Design review of the part built by this model. Coordinates are the model's own, in mm. A direction names the side the tool comes from. Round coordinates to 2 decimals unless told otherwise and drop trailing zeros. Loops run counter-clockwise (first coordinate to the right, second up) from the corner with the lowest first, then second, coordinate; pieces in that order, holes last. Notation, with made-up numbers: M 18.5,88.5 L 31.5,88.5 A25 cw 31.5,104.5 Z; hole C 87,-17.5 d6. An arc over 180 degrees is marked long. One line per item, written item: value. Start each with the question number.
Item 1: We need section D-D (x = -87.5). Write out the cut boundary in (y, z), then the cut area to 3 significant figures.
Item 2: For line 1 along Y through (x, z) = (37.5, 6); line 2 along Y through (x, z) = (20.5, 1); line 3 along Y through (x, z) = (-58, 1.25), list the stretches that pass through material, from the lowest coordinate up.
Item 3: Clearance check with flat-ended pins moving along their axes: pin 1 (1.5 mm diameter, centred on y = -19, z = 2.5, fed in from +X); pin 2 (2.5 mm diameter, centred on x = 44.5, z = 4.5, fed in from -Y); pin 3 (2.5 mm diameter, centred on x = -53, z = 2.5, fed in from -Y); pin 4 (5.5 mm diameter, centred on x = -37.5, y = -37.5, fed in from +Z). State where each tip first meets the part, or that it passes through.
Item 4: We need section A-A (x = -8). Write out the cut boundary in (y, z).
Item 5: We need section C-C (z = 2.75). State how many separate pieces and enclosed holes the cut face has, then the cut area to 3 significant figures.
Item 6: Mouldability with a two-part tool opening along Y and no side actions: class faces 1 (the cylindrical face through (50.35, 23.01, 4.06)), 2 (the flat face through (-47.5, -34, 4)), 3 (the flat face through (0, 27.5, 4)) as released by +Y, released by -Y, zero draft, split by the parting line, or undercut.
Item 7: We need section B-B (y = 0). Write out the cut boundary in (x, z), then the cut area to 3 significant figures.
Item 8: For faces 4 (the cylindrical face through (50.51, -22.85, 4.06)), 5 (the flat face through (65, 0, 4)), list the 3-axis set-ups (+Z, -Z, +X, -X, +Y, -Y) from which the entire face can be reached by the end or side of a thin tool; tool diameter is ignored.
Autodesk Inventor part; units mm, degrees
ref_plane "YZ Plane" through (0, 0, 0) normal (1, 0, 0) x (0, 1, 0)
ref_plane "XZ Plane" through (0, 0, 0) normal (0, 1, 0) x (-1, 0, 0)
ref_plane "XY Plane" through (0, 0, 0) normal (0, 0, 1) x (1, 0, 0)
sketch "Sketch1" plane through (0, 0, 0) normal (0, 0, 1) x (1, 0, 0)
  line L0 (-50, -50) -> (50, -50) construction
  line L1 (50, -50) -> (50, 50) construction
  line L2 (50, 50) -> (-50, 50) construction
  line L3 (-50, 50) -> (-50, -50) construction
  line L4 (-50, -50) -> (50, 50) construction
  line L5 (50, -50) -> (-50, 50) construction
  line L6 (-37.5, -37.5) -> (37.5, -37.5) construction
  line L7 (37.5, -37.5) -> (37.5, 37.5) construction
  line L8 (37.5, 37.5) -> (-37.5, 37.5) construction
  line L9 (-37.5, 37.5) -> (-37.5, -37.5) construction
  line L10 (-37.5, -37.5) -> (37.5, 37.5) construction
  line L11 (37.5, -37.5) -> (-37.5, 37.5) construction
  line L12 (-47.5, -47.5) -> (47.5, -47.5)
  line L13 (47.5, -47.5) -> (47.5, 47.5)
  line L14 (47.5, 47.5) -> (-47.5, 47.5)
  line L15 (-47.5, 47.5) -> (-47.5, -47.5)
  line L16 (-47.5, -47.5) -> (47.5, 47.5) construction
  line L17 (47.5, -47.5) -> (-47.5, 47.5) construction
  circle A0 centre (-50, 50) radius 2.15
  circle A1 centre (-37.5, 37.5) radius 2.15
  circle A2 centre (37.5, 37.5) radius 2.15
  circle A3 centre (-37.5, -37.5) radius 2.15
  circle A4 centre (37.5, -37.5) radius 2.15
  circle A5 centre (50, 50) radius 2.15
  circle A6 centre (-50, -50) radius 2.15
  circle A7 centre (50, -50) radius 2.15
  line L18 (-95, -20) -> (95, -20)
  line L19 (95, -20) -> (95, 20)
  line L20 (95, 20) -> (-95, 20)
  line L21 (-95, 20) -> (-95, -20)
  line L22 (-95, -20) -> (95, 20) construction
  line L23 (95, -20) -> (-95, 20) construction
  circle A8 centre (87.5, 0) radius 2.15
  line L24 (0, 0) -> (0, 12.464) construction
  circle A9 centre (-87.5, 0) radius 2.15
  point P0 (-47.5, -20)
  point P1 (-47.5, 20)
  point P2 (47.5, 20)
  point P3 (47.5, -20)
  dimension "d0" = 100
  dimension "d1" = 100
  dimension "d2" = 75
  dimension "d3" = 75
  dimension "d4" = 95
  dimension "d5" = 95
  dimension "d6" = 4.3
  dimension "d7" = 4.3
  dimension "d10" = 75
  dimension "d13" = 75
  dimension "d18" = 100
  dimension "d21" = 100
  dimension "d31" = 40
  dimension "d32" = 4.3
  dimension "d33" = 87.5
  dimension "d34" = 7.5
extrude "Extrusion1" add sketch "Sketch1" along normal blind 8 contours L15 L18 L13 L12 | L18 L21 L20 L15 | L15 L20 L13 L18 | L13 L20 L19 L18 | L15 L14 L13 L20
sketch "Sketch3" plane through (0, 0, 8) normal (0, 0, 1) x (1, 0, 0)
  line L0 (47.5, 47.5) -> (-47.5, 47.5)
  line L1 (-47.5, 47.5) -> (-47.5, 20)
  line L2 (-47.5, 20) -> (-95, 20)
  line L3 (-95, 20) -> (-95, -20)
  line L4 (-95, -20) -> (-47.5, -20)
  line L5 (-47.5, -20) -> (-47.5, -47.5)
  line L6 (-47.5, -47.5) -> (47.5, -47.5)
  line L7 (47.5, -47.5) -> (47.5, -20)
  line L8 (47.5, -20) -> (95, -20)
  line L9 (95, -20) -> (95, 20)
  line L10 (95, 20) -> (47.5, 20)
  line L11 (47.5, 20) -> (47.5, 47.5)
  line L12 (-27.5, -27.5) -> (27.5, -27.5)
  line L13 (27.5, -27.5) -> (27.5, 27.5)
  line L14 (27.5, 27.5) -> (-27.5, 27.5)
  line L15 (-27.5, 27.5) -> (-27.5, -27.5)
  line L16 (-27.5, -27.5) -> (27.5, 27.5) construction
  line L17 (27.5, -27.5) -> (-27.5, 27.5) construction
  line L18 (-65, -7.5) -> (65, -7.5)
  line L19 (65, -7.5) -> (65, 7.5)
  line L20 (65, 7.5) -> (-65, 7.5)
  line L21 (-65, 7.5) -> (-65, -7.5)
  line L22 (-65, -7.5) -> (65, 7.5) construction
  line L23 (65, -7.5) -> (-65, 7.5) construction
  point P0 (0, 0)
  point P1 (-27.5, 7.5)
  point P2 (-27.5, -7.5)
  point P3 (27.5, -7.5)
  point P4 (27.5, 7.5)
  dimension "d35" = 55
  dimension "d36" = 55
  dimension "d37" = 130
  dimension "d38" = 15
extrude "Extrusion3" cut sketch "Sketch3" against normal through all contours L15 L18 L13 L12 | L18 L21 L20 L15 | L15 L20 L13 L18 | L13 L20 L19 L18 | L15 L14 L13 L20
fillet "Fillet1" radius 10 16 edges at (-47.5, -47.5, 4) (-47.5, -20, 4) (-95, -20, 4) (-47.5, 47.5, 4) (-95, 20, 4) (47.5, 47.5, 4) (95, 20, 4) (47.5, 20, 4) (95, -20, 4) (47.5, -20, 4) (47.5, -47.5, 4) (-47.5, 20, 4) (27.5, -7.5, 4) (27.5, 7.5, 4) (-27.5, 7.5, 4) (-27.5, -7.5, 4)
fillet "Fillet1" radius 5 8 edges at (27.5, 27.5, 4) (65, 7.5, 4) (65, -7.5, 4) (27.5, -27.5, 4) (-27.5, -27.5, 4) (-27.5, 27.5, 4) (-65, -7.5, 4) (-65, 7.5, 4)
equation "\"d1\" = d0"
equation "\"d5\" = d4"
equation "\"d35\" = d36"
properties part number "Power_box"
A:
1. outline: M -19.68,0 L -2.15,0 L -2.15,8 L -19.68,8 Z; M 2.15,0 L 19.68,0 L 19.68,8 L 2.15,8 Z
1. area: 281 mm2
2. line 1: -47.5 to -39.65, -35.35 to -7.5, 7.5 to 35.35, 39.65 to 47.5
2. line 2: -47.5 to -27.5, 27.5 to 47.5
2. line 3: -20 to -7.5, 7.5 to 20
3. pin 1: x = 90.65
3. pin 2: y = -45.68
3. pin 3: y = -21.82
3. pin 4: z = 8
4. outline: M -47.5,0 L -27.5,0 L -27.5,8 L -47.5,8 Z; M 27.5,0 L 47.5,0 L 47.5,8 L 27.5,8 Z
5. separate pieces: 1
5. enclosed holes: 7
5. area: 8,460 mm2
6. face 1: released by +Y
6. face 2: zero draft
6. face 3: undercut
7. outline: M -95,0 L -89.65,0 L -89.65,8 L -95,8 Z; M -85.35,0 L -65,0 L -65,8 L -85.35,8 Z; M 65,0 L 85.35,0 L 85.35,8 L 65,8 Z; M 89.65,0 L 95,0 L 95,8 L 89.65,8 Z
7. area: 411 mm2
8. face 4: +Z, -Z, +X, -Y
8. face 5: +Z, -Z
